```python
from build123d import *

# Parameters (mm, degrees)
SKETCH1_R                = 58.166
BOSS_EXTRUDE1_DEPTH      = 21.971
SKETCH3_R                = 51.816
CUT_EXTRUDE2_DEPTH       = 18.796
CUT_EXTRUDE7_DEPTH       = 18.796
SKETCH7_R                = 6.477
BOSS_EXTRUDE3_DEPTH      = 11.43
BOSS_EXTRUDE3_DEPTH_BACK = 10.9855


with BuildPart() as part:
    # Sketch1 → Boss-Extrude1 (new body)
    with BuildSketch(Plane(origin=(0, 0, 0), x_dir=(1, 0, 0), z_dir=(0, 1, 0))):
        Circle(SKETCH1_R)
    extrude(amount=BOSS_EXTRUDE1_DEPTH)

    # Sketch3 → Cut-Extrude2 (cut)
    with BuildSketch(Plane(origin=(0, 21.971, 0), x_dir=(1, 0, 0), z_dir=(0, 1, 0))):
        Circle(SKETCH3_R)
    extrude(amount=-CUT_EXTRUDE2_DEPTH, mode=Mode.SUBTRACT)

    # Sketch6 → Cut-Extrude7 (cut)
    with BuildSketch(Plane(origin=(0, 21.971, 0), x_dir=(1, 0, 0), z_dir=(0, 1, 0))):
        with BuildLine():
            Line((9.363048829, 50.963037318), (9.340756891, 57.411094892))
            ThreePointArc((9.340756891, 57.411094892), (2.903170649, 58.093503563), (-3.57037671, 58.056317194))
            Line((-3.57037671, 58.056317194), (-3.57037671, 51.692845406))
            ThreePointArc((-3.57037671, 51.692845406), (2.919232353, 51.733702153), (9.363048829, 50.963037318))
        make_face()
    extrude(amount=-CUT_EXTRUDE7_DEPTH, mode=Mode.SUBTRACT)

    # Sketch7 → Boss-Extrude3 (add, two sides)
    with BuildSketch(Plane.XZ) as boss_extrude3_sk:
        with BuildLine():
            ThreePointArc((55.382885714, -17.776938037), (81.28, 0), (55.382885714, 17.776938037))
            ThreePointArc((55.382885714, 17.776938037), (58.166, 0), (55.382885714, -17.776938037))
        make_face()
        with Locations((68.326, 0)):
            Circle(SKETCH7_R, mode=Mode.SUBTRACT)
        with BuildLine():
            ThreePointArc((-55.382885714, 17.776938037), (-81.28, 0), (-55.382885714, -17.776938037))
            ThreePointArc((-55.382885714, -17.776938037), (-58.166, 0), (-55.382885714, 17.776938037))
        make_face()
        with Locations((-68.323824172, 0)):
            Circle(SKETCH7_R, mode=Mode.SUBTRACT)
    extrude(amount=BOSS_EXTRUDE3_DEPTH)
    extrude(boss_extrude3_sk.sketch, amount=-BOSS_EXTRUDE3_DEPTH_BACK)


solid = part.part
```
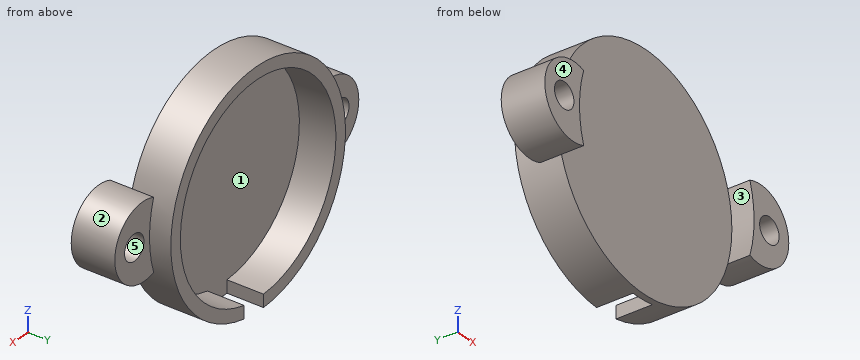
The listing builds one solid part. Answer for the finished solid, in the listing's coordinates (mm). Face numbers are marked on the shaded views. A direction names the side the tool comes from. Give positions to 0.01 mm unless a question says otherwise; leave off trailing zeros. Loops run counter-clockwise (first coordinate to the right, second up) from the corner with the lowest first, then second, coordinate; pieces in that order, holes last. Notation, with made-up numbers: (-38.75, 86.5) - (-0.75, 86.5) arc R27 cw to (-0.75, 110.5) - close; hole circle Ø7 at (16.5, 23). An arc over 180 degrees is marked (long way). Return JSON: item names as keys, results as strings. Group by question number.
1. Find section C-C (x = 70). Write down the section's boundary in (y, z).
2. Determine the mould class of the marked faces 4 and 5 for opening direction X: pulls with the +X half, pulls with the -X half, needs draft (parallel to the pull), parting line crosses it, or undercut.
3. Find section D-D (z = 28). Write down the section's boundary in (x, y) (3 decimals).
4. Find section B-B (z = 0). Write down the section's boundary in (x, y) (1 decimal), then the cut area to 3 significant figures.
5. Find section A-A (y = -7.5). Write down the section's boundary in (x, z).
6. Straight lines are drawn through the part: line 1 (X direction, y = 11.5, z = 0); line 2 (X direction, y = 8, z = 2); line 3 (Y direction, x = -55, z = 1.5). For each, find the intervals that lie inside material, in ascending order. Write a range as [from, to].
7. Given pin 1 Ø20.5 at (x, z) = (73.5, -2.5) entering from +Y; pin 2 Ø8 at (x, y) = (20.5, -7.5) entering from -Z; pin 3 Ø3 at (x, y) = (-50, 18) entering from -Z; pin 4 Ø4 at (x, y) = (32.5, 3.5) entering from +Z, each flat-ended and moving along its own axis, determine where each tip first touches the part or whether it passes through.
8. Which of the six approach directions +Z, -Z, +X, -X, +Y, -Y give full straight-line access (tool end or side, diameter ignored) to the marked faces 1, 2 and 3?
Verdict:
{
 "1": {"outline": "(-11.43, -17.39) - (10.99, -17.39) - (10.99, -6.26) - (-11.43, -6.26) - close; (-11.43, 6.26) - (10.99, 6.26) - (10.99, 17.39) - (-11.43, 17.39) - close"},
 "2": {"face 4": "needs draft", "face 5": "undercut"},
 "3": {"outline": "(-50.983, 0) - (50.983, 0) - (50.983, 21.971) - (43.599, 21.971) - (43.599, 3.175) - (-43.599, 3.175) - (-43.599, 21.971) - (-50.983, 21.971) - close"},
 "4": {"outline": "(-81.3, -11.4) - (-74.8, -11.4) - (-74.8, 11) - (-81.3, 11) - close; (-61.8, -11.4) - (-58.2, -11.4) - (-58.2, 0) - (58.2, 0) - (58.2, -11.4) - (61.8, -11.4) - (61.8, 11) - (58.2, 11) - (58.2, 22) - (51.8, 22) - (51.8, 3.2) - (-51.8, 3.2) - (-51.8, 22) - (-58.2, 22) - (-58.2, 11) - (-61.8, 11) - close; (74.8, -11.4) - (81.3, -11.4) - (81.3, 11) - (74.8, 11) - close", "area": "1,060 mm^2"},
 "5": {"outline": "(-55.38, -17.78) arc R58.17 cw to (-55.38, 17.78) arc R19.05 ccw (long way) to start; (55.38, -17.78) arc R19.05 ccw (long way) to (55.38, 17.78) arc R58.17 cw to start; hole circle Ø12.95 at (-68.32, 0); hole circle Ø12.95 at (68.33, 0)"},
 "6": {"line 1": "x = [-58.17, -51.82], [51.82, 58.17]", "line 2": "x = [-81.17, -74.48], [-62.16, -51.78], [51.78, 62.17], [74.49, 81.17]", "line 3": "y = [0, 21.97]"},
 "7": {"pin 1": "stops at y = 10.99", "pin 2": "passes through", "pin 3": "stops at z = -32.11", "pin 4": "stops at z = 49.53"},
 "8": {"face 1": "+Y", "face 2": "+Y, -Y", "face 3": "-Y"}
}
